Autodesk Inventor part; units mm, degrees
ref_plane "YZ Plane" through (0, 0, 0) normal (1, 0, 0) x (0, 1, 0)
ref_plane "XZ Plane" through (0, 0, 0) normal (0, 1, 0) x (-1, 0, 0)
ref_plane "XY Plane" through (0, 0, 0) normal (0, 0, 1) x (1, 0, 0)
sketch "Sketch1" plane through (0, 0, 0) normal (1, 0, 0) x (0, 1, 0)
  line L0 (-12.7, 12.7) -> (12.7, 12.7)
  line L1 (12.7, 12.7) -> (12.7, -12.7)
  line L2 (12.7, -12.7) -> (-12.7, -12.7)
  line L3 (-12.7, -12.7) -> (-12.7, 12.7)
  line L4 (-11.1125, 11.1125) -> (11.1125, 11.1125)
  line L5 (11.1125, 11.1125) -> (11.1125, -10.8514)
  line L6 (11.1125, -10.8514) -> (-11.1125, -10.8514)
  line L7 (-11.1125, -10.8514) -> (-11.1125, 11.1125)
  point P0 (0, 0)
  point P1 (0, 12.7)
  point P2 (-12.7, 0)
  dimension "d0" = 25.4
  dimension "d1" = 25.4
  dimension "d2" = 1.5875
  dimension "d3" = 1.5875
  dimension "d4" = 1.5875
extrude "Extrusion1" add sketch "Sketch1" along normal blind 787.4
sketch "Sketch2" plane through (0, -12.7, 12.7) normal (0, 0, 1) x (1, 0, 0)
  circle A0 centre (9.525, 12.7) radius 6.35
  circle A1 centre (777.875, 12.7) radius 6.35
  line L0 (787.4, 25.4) -> (787.4, 0)
  point P0 (0, 12.7)
  dimension "d7" = 12.7
  dimension "d8" = 9.525
  dimension "d9" = 12.7
  dimension "d10" = 9.525
extrude "Extrusion2" cut sketch "Sketch2" against normal blind 50.8
equation "\"d1\" = d0"
equation "\"d3\" = d2"
equation "\"d4\" = d2"
equation "\"d9\" = d7"
equation "\"d10\" = d8"
properties part number "Long Bar"
Geometry: final body of the model. Coordinates: model frame, mm. A direction names the side the tool comes from. Give positions to 0.01 mm unless a question says otherwise; leave off trailing zeros. Write each loop counter-clockwise with the first axis right and the second up, starting at its lowest first coordinate (ties: lowest second). Pieces come first, ordered by that corner, then holes. Notation, with made-up numbers: (81, 23) - (97, 23) arc R25 cw to (97, 59) - close; hole circle Ø10 at (-7, -5). An arc over 180 degrees is marked (long way). Return JSON: item names as keys, results as strings. Group by question number.
1) Section B-B on x = 603. Return the cut outline in (y, z).
2) Section C-C on z = 3.5. Return the cut outline in (x, y), plus the area to 3 significant figures.
3) Mould query, pull axis Y, two halves, no side actions, for faces 3 (the flat face through (388, 0, -10.851)), 4 (the flat face through (388, 12.7, 0)), 5 (the flat face through (388, -12.7, 0)). Classes: released by +Y, released by -Y, zero draft, split by the parting line, or undercut.
4) Line query: line 1 (Z direction, x = 311, y = -10.25); line 2 (Y direction, x = 325, z = 10.25); line 3 (X direction, y = 4.5, z = -11.25). Output: solid intervals per line, ascending.
5) Set-up query: faces 1 (the flat face through (388, 11.112, 0)), 2 (the cylindrical face through (783.93, 1.91, -11.76)). Return all of +Z, -Z, +X, -X, +Y, -Y with unobstructed straight access to the full face (end or side cutting, diameter ignored); none if empty.
6) Section A-A on y = 0. Return the cut outline in (x, z) (1 decimal), plus the area to 3 significant figures.
Filled in:
{
 "1": {"outline": "(-12.7, -12.7) - (12.7, -12.7) - (12.7, 12.7) - (-12.7, 12.7) - close; hole (-11.11, -10.85) - (11.11, -10.85) - (11.11, 11.11) - (-11.11, 11.11) - close"},
 "2": {"outline": "(0, -12.7) - (787.4, -12.7) - (787.4, -11.11) - (0, -11.11) - close; (0, 11.11) - (787.4, 11.11) - (787.4, 12.7) - (0, 12.7) - close", "area": "2,500 mm^2"},
 "3": {"face 3": "undercut", "face 4": "released by +Y", "face 5": "released by -Y"},
 "4": {"line 1": "z = -12.7 to -10.85, 11.11 to 12.7", "line 2": "y = -12.7 to -11.11, 11.11 to 12.7", "line 3": "x = 0 to 5.04, 14.01 to 773.39, 782.36 to 787.4"},
 "5": {"face 1": "+X, -X", "face 2": "+Z, -Z"},
 "6": {"outline": "(0, -12.7) - (3.2, -12.7) - (3.2, -10.9) - (0, -10.9) - close; (0, 11.1) - (3.2, 11.1) - (3.2, 12.7) - (0, 12.7) - close; (15.9, -12.7) - (771.5, -12.7) - (771.5, -10.9) - (15.9, -10.9) - close; (15.9, 11.1) - (771.5, 11.1) - (771.5, 12.7) - (15.9, 12.7) - close; (784.2, -12.7) - (787.4, -12.7) - (787.4, -10.9) - (784.2, -10.9) - close; (784.2, 11.1) - (787.4, 11.1) - (787.4, 12.7) - (784.2, 12.7) - close", "area": "2,620 mm^2"}
}
